Can you work these out from the model? Positions are in its coordinate system, mm. A direction names the side the tool comes from. Coordinates: 2 decimals unless noted, no trailing zeros. Order: outer loops, then holes, each group sorted by start corner. A loop starts at its lowest first (then second) coordinate and runs counter-clockwise, first axis right, second up. Notation, with made-up numbers: M -13.5,-16 L 35.5,-16 A16 ccw 35.5,11 Z; hole C 19,68 d11. An arc over 180 degrees is marked long. Answer as a JSON object with one key per item and string values.
from build123d import *

# Parameters (mm, degrees)
F1_DEPTH = 76.2
F3_DEPTH = 38.1


with BuildPart() as f1:
    # F0 (on Top) → F1 (new body)
    with BuildSketch(Plane.XY):
        Polygon((-838.2, 457.2), (-838.2, -1066.8), (-762, -1066.8), (-762, 381), (762, 381), (762, -1066.8), (838.2, -1066.8), (838.2, 457.2), align=None)
    extrude(amount=F1_DEPTH)

    # F2 (on Right) → F3 (join, symmetric)
    with BuildSketch(Plane.YZ):
        Polygon((381, 0), (457.2, 0), (457.2, 76.2), (587.509675, 434.222889), (587.509675, 1450.222889), (206.509675, 1450.222889), (206.509675, 1374.022889), (511.309675, 1374.022889), (511.309675, 434.222889), (381, 76.2), align=None)
    extrude(amount=F3_DEPTH, both=True)


solid = f1.part
Item 1: If we mould it in two halves opening along Z, with no side actions, what happens to faces 6 (the flat face through (1, 357, 1374.023)), 7 (the flat face through (1, 511.31, 911)), 8 (the flat face through (0.533, 521.443, 252.705)), 9 (the flat face through (762, -333, 38))? For each: pulls with the +Z half, pulls with the -Z half, needs draft (parallel to the pull), parting line crosses it, or undercut.
Answers follow:
{"face 6": "undercut", "face 7": "undercut", "face 8": "pulls with the -Z half", "face 9": "needs draft"}
Item 2: Which directions (+Z, -Z, +X, -X, +Y, -Y) give clear straight access to the entire face, cutting with the end or side of a thin tool? Please do faces 1 (the flat face through (762.2, -131.9, 76.2)), 2 (the flat face through (-766, -132, 76.2)), 3 (the flat face through (-762, -353, 38)), 4 (the flat face through (0.53, 447.07, 257.72)), 5 (the flat face through (1, 206.51, 1413)).
Answers follow:
{"face 1": "+Z, +X, +Y, -Y", "face 2": "+Z, -X, +Y, -Y", "face 3": "+Z, -Z, -Y", "face 4": "+X, -X, -Y", "face 5": "+Z, -Z, +X, -X, -Y"}
Item 3: I want a section at A-A, the plane y = -267.5. Write out the boundary of the cut face in (x, z), plus the area to 3 significant figures.
Answers follow:
{"outline": "M -838.2,0 L -762,0 L -762,76.2 L -838.2,76.2 Z; M 762,0 L 838.2,0 L 838.2,76.2 L 762,76.2 Z", "area": "11,600 mm^2"}
Item 4: I'm going to push a flat-ended pin straight in: pin 1 (23 mm diameter, centred on x = -104, z = 32, fed in from -Y). Where does the tip first touch, or does it pass through?
Answers follow:
{"pin 1": "stops at y = 381"}
Item 5: Please list where these lines run through material, in increasing order: line 1 (Z direction, x = 9.5, y = 216); line 2 (Z direction, x = -574, y = 442).
Answers follow:
{"line 1": "z = 1374.02 to 1450.22", "line 2": "z = 0 to 76.2"}
Item 6: I want a section at B-B, the plane x = -268.5. Write out the boundary of the cut face in (y, z).
Answers follow:
{"outline": "M 381,0 L 457.2,0 L 457.2,76.2 L 381,76.2 Z"}
Item 7: I want a section at C-C, the plane z = 114.5. Write out the boundary of the cut face in (x, y), plus the area to 3 significant figures.
Answers follow:
{"outline": "M -38.1,394.94 L 38.1,394.94 L 38.1,471.14 L -38.1,471.14 Z", "area": "5,810 mm^2"}
